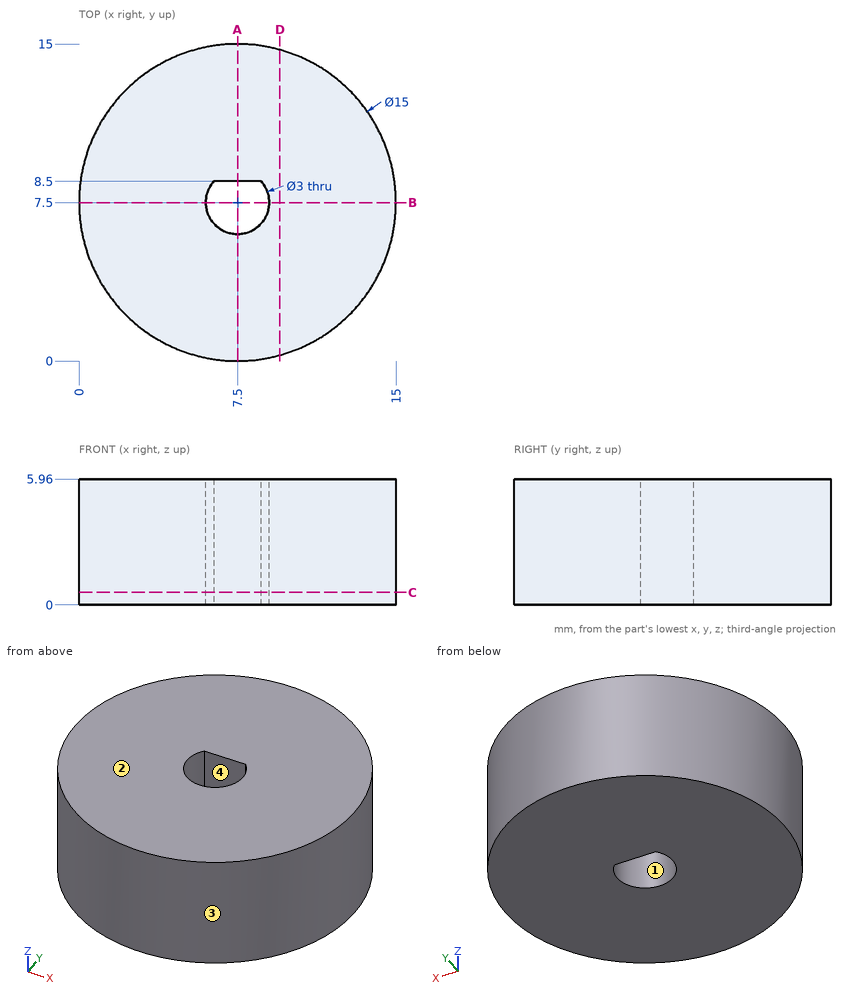
The figure shows three views and two pictorial views of one solid part (mm, origin at its lowest corner). Answer the questions. Coordinates: 2 decimals unless noted, no trailing zeros. Loops run counter-clockwise (first coordinate to the right, second up) from the corner with the lowest first, then second, coordinate; pieces in that order, holes last. Notation, with made-up numbers: (58, 34) - (98, 34) arc R13 ccw to (98, 50) - close; hole circle Ø4 at (63, 18.25). An arc over 180 degrees is marked (long way). Write item = value, one per line.
1) Section C-C (z = 0.6) is taken. Determine the outline of the cut face in (x, y).
Responses:
outline = circle Ø15 at (7.5, 7.5); hole (6.38, 8.5) arc R1.5 ccw (long way) to (8.62, 8.5) - close
2) Section D-D (x = 9.5) is taken. Determine the outline of the cut face in (y, z).
Responses:
outline = (0.27, 0) - (14.73, 0) - (14.73, 5.96) - (0.27, 5.96) - close
3) Section A-A (x = 7.5) is taken. Determine the outline of the cut face in (y, z).
Responses:
outline = (0, 0) - (6, 0) - (6, 5.96) - (0, 5.96) - close; (8.5, 0) - (15, 0) - (15, 5.96) - (8.5, 5.96) - close
4) Each of these flat-tipped pins is pushed along its axis until it touches: P1, Ø2, axis at x = 4, z = 1.5, coming from the -Y side; P2, Ø1.5, axis at y = 13, z = 0.5, coming from the +X side. Where does it stop, or does it pass through?
Responses:
P1 = 0.43
P2 = 13.3
5) Section B-B (y = 7.5) is taken. Determine the outline of the cut face in (x, z).
Responses:
outline = (0, 0) - (6, 0) - (6, 5.96) - (0, 5.96) - close; (9, 0) - (15, 0) - (15, 5.96) - (9, 5.96) - close
6) Find the intervals of material crossed by line 1 along Y through (x, z) = (7.5, 2.35); line 2 along Y through (x, z) = (6.5, 5.35); line 3 along X through (y, z) = (3.5, 2.75), in increasing order.
Responses:
line_1 = 0 to 6, 8.5 to 15
line_2 = 0.07 to 6.38, 8.5 to 14.93
line_3 = 1.16 to 13.84
7) Determine the mould class of the marked faces 1, 2, 3 and 4 for opening direction X: pulls with the +X half, pulls with the -X half, needs draft (parallel to the pull), parting line crosses it, or undercut.
Responses:
face_1 = undercut
face_2 = needs draft
face_3 = parting line crosses it
face_4 = undercut
